The drawing under review shows one solid part. Ordinate dimensions are in mm from its lowest x, y, z. A direction names the side the tool comes from. Give positions to 0.01 mm unless a question says otherwise; leave off trailing zeros. Order: outer loops, then holes, each group sorted by start corner. A loop starts at its lowest first (then second) coordinate and runs counter-clockwise, first axis right, second up. Notation, with made-up numbers: (47, 15.5) - (106, 15.5) arc R30 ccw to (106, 47.5) - close; hole circle Ø10 at (84, 36.25). An arc over 180 degrees is marked (long way). Use CSV: the item, a comma, the result in double quotes. Start each with the question number.
1. Draft analysis for pull direction X (two halves, no side actions). For the marked faces 3, 4 and 5, state which applies: released by +X, released by -X, zero draft, split by the parting line, or undercut.
2. Take a section at A-A, the plane z = 5.25. State the section outline as (x, y) points, then the cut area to 3 significant figures.
3. Take a section at B-B, the plane x = 21.5. State the section outline as (y, z) points.
4. Machinability: for the marked faces 1 and 2, which of the approach directions +Z, -Z, +X, -X, +Y, -Y give a long, thin tool a straight path to every point of the face, cutting with its end or side? Answer none if there is none.
5. To check wall thickness, follow line 1 (X direction, y = 8.5, z = 20); line 2 (Y direction, x = 24, z = 15.25). State the ranges of each line that lie inside material, in increasing order. Write a range as [from, to].
6. For pin 1 (1 mm diameter, centred on x = 30, y = 16, fed in from -Z), flat-tipped, find the tip position at first contact; note if it passes through.
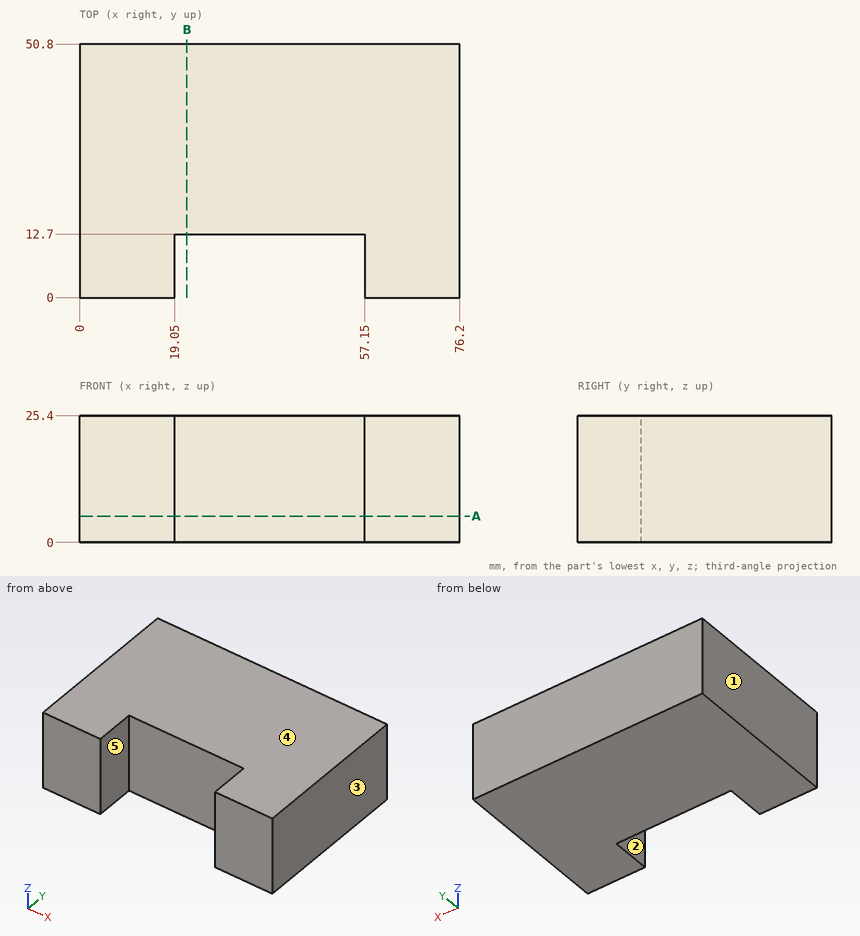
Determined:
1,face 3,"released by +X"
1,face 4,"zero draft"
1,face 5,"undercut"
2,outline,"(0, 0) - (19.05, 0) - (19.05, 12.7) - (57.15, 12.7) - (57.15, 0) - (76.2, 0) - (76.2, 50.8) - (0, 50.8) - close"
2,area,"3,390 mm²"
3,outline,"(12.7, 0) - (50.8, 0) - (50.8, 25.4) - (12.7, 25.4) - close"
4,face 1,"+Z, -Z, -X, +Y, -Y"
4,face 2,"+Z, -Z, -Y"
5,line 1,"x = [0, 19.05], [57.15, 76.2]"
5,line 2,"y = [12.7, 50.8]"
6,pin 1,"stops at z = 0"
